from build123d import *

# Parameters (mm, degrees)
SKETCH1_W           = 111.5
SKETCH1_H           = 75
BOSS_EXTRUDE1_DEPTH = 63
CUT_EXTRUDE1_REACH  = 114.703
SKETCH3_W           = 22
SKETCH3_H           = 7
CUT_EXTRUDE2_DEPTH  = 15
CUT_EXTRUDE3_DEPTH  = 15
FILLET1_R           = 10
FILLET2_R           = 2


with BuildPart() as part:
    # Sketch1 → Boss-Extrude1 (new body)
    with BuildSketch(Plane(origin=(0, 0, 0), x_dir=(1, 0, 0), z_dir=(0, 1, 0))):
        Rectangle(SKETCH1_W, SKETCH1_H)
    extrude(amount=BOSS_EXTRUDE1_DEPTH)

    # Sketch2 → Cut-Extrude1 (cut, up to next)
    with BuildSketch(Plane.XY.offset(37.5), mode=Mode.PRIVATE) as cut_extrude1_sk1:
        Polygon((-55.75, 41), (-33.75, 63), (-55.75, 63), align=None)
    cut_extrude1_tool1 = extrude(cut_extrude1_sk1.sketch, amount=-CUT_EXTRUDE1_REACH, mode=Mode.PRIVATE) & part.part
    # Sketch2 → Cut-Extrude1 (cut, up to next)
    with BuildSketch(Plane.XY.offset(37.5), mode=Mode.PRIVATE) as cut_extrude1_sk2:
        Polygon((-55.75, 15), (-40.75, 0), (-55.75, 0), align=None)
    cut_extrude1_tool2 = extrude(cut_extrude1_sk2.sketch, amount=-CUT_EXTRUDE1_REACH, mode=Mode.PRIVATE) & part.part
    add(cut_extrude1_tool1.solids().sort_by_distance((-48.416667, 55.666667, 37.5))[0], mode=Mode.SUBTRACT)
    add(cut_extrude1_tool2.solids().sort_by_distance((-50.75, 5, 37.5))[0], mode=Mode.SUBTRACT)

    # Sketch3 → Cut-Extrude2 (cut)
    with BuildSketch(Plane(origin=(0, 63, 0), x_dir=(1, 0, 0), z_dir=(0, 1, 0))):
        Polygon((31.25, -30.5), (-33.75, -30.5), (-33.75, -37.5), (55.75, -37.5), (55.75, 37.5), (-33.75, 37.5), (-33.75, 30.5), (31.25, 30.5), align=None)
        with Locations((-44.75, -34)):
            Rectangle(SKETCH3_W, SKETCH3_H)
        with Locations((-44.75, 34)):
            Rectangle(SKETCH3_W, SKETCH3_H)
    extrude(amount=-CUT_EXTRUDE2_DEPTH, mode=Mode.SUBTRACT)

    # Sketch4 → Cut-Extrude3 (cut, symmetric)
    with BuildSketch(Plane.XY):
        Polygon((-53.628679656, 43.121320344), (-38.699747468, 58.050252532), (-38.699747468, 55.221825407), (-50.800252532, 43.121320344), align=None)
    extrude(amount=CUT_EXTRUDE3_DEPTH, both=True, mode=Mode.SUBTRACT)

    # Fillet1
    # the kernel refuses this fillet: 10 mm, written as the material it takes off along each edge
    with BuildSketch(Plane(origin=(-55.75, 41, 47.855339059), x_dir=(0.7071067811865432, 0.7071067811865519, 0), z_dir=(0, 0, -1)), Plane(origin=(-40.75, 0, 47.855339059), x_dir=(-0.707106781186546, 0.707106781186549, 0), z_dir=(0, 0, -1))) as fillet1_piece_1:
        with BuildLine():
            CenterArc((FILLET1_R * 0.414213562373, FILLET1_R), FILLET1_R, 225, 45)
            Line((-FILLET1_R * 0.292893218813, FILLET1_R * 0.292893218813), (0, 0))
            Line((0, 0), (FILLET1_R * 0.414213562373, 0))
        make_face()
    extrude(amount=95.710678119, mode=Mode.SUBTRACT)
    with BuildSketch(Plane(origin=(-55.75, 15, 47.855339059), x_dir=(0.7071067811865466, -0.7071067811865482, 0), z_dir=(0, 0, -1))) as fillet1_piece_2:
        with BuildLine():
            CenterArc((FILLET1_R * 0.414213562373, -FILLET1_R), FILLET1_R, 90, 45)
            Line((-FILLET1_R * 0.292893218813, -FILLET1_R * 0.292893218813), (0, 0))
            Line((0, 0), (FILLET1_R * 0.414213562373, 0))
        make_face()
    extrude(amount=95.710678119, mode=Mode.SUBTRACT)
    with BuildSketch(Plane(origin=(55.75, 0, -62.5), x_dir=(-1, 0, 0), z_dir=(0, 0, 1))) as fillet1_piece_3:
        with BuildLine():
            CenterArc((FILLET1_R, -FILLET1_R), FILLET1_R, 90, 90)
            Line((0, -FILLET1_R), (0, 0))
            Line((0, 0), (FILLET1_R, 0))
        make_face()
    extrude(amount=125, mode=Mode.SUBTRACT)

    # Fillet2
    fillet2_edges = [part.edges().sort_by_distance(p)[0] for p in [
        (4.571067812, 0, -37.5),
        (-48.25, 7.5, -37.5),
        (52.821067812, 2.928932188, -37.5),
        (-40.4346987, 0.761204675, -37.5),
        (-54.988795325, 15.3153013, -37.5),
        (-54.988795325, 40.6846987, -37.5),
        (-50.785533906, 45.964466094, -37.5),
        (55.75, 29, 37.5),
        (55.75, 29, -37.5),
        (3.5, 48, -37.5),
        (3.5, 48, 37.5),
        (55.75, 48, 0),
        (-50.785533906, 45.964466094, 37.5),
        (-55.75, 28, 37.5),
        (-48.25, 7.5, 37.5),
        (4.571067812, 0, 37.5),
        (52.821067812, 2.928932188, 37.5),
        (-40.4346987, 0.761204675, 37.5),
        (-54.988795325, 15.3153013, 37.5),
        (-54.988795325, 40.6846987, 37.5),
        (-55.75, 28, -37.5),
    ]]
    fillet(fillet2_edges, radius=FILLET2_R)


solid = part.part
Model file for the job. Use its own axes, mm. A direction names the side the tool comes from. Coordinates: 2 decimals unless noted, no trailing zeros. Write each loop counter-clockwise with the first axis right and the second up, starting at its lowest first coordinate (ties: lowest second). Pieces come first, ordered by that corner, then holes. Notation, with made-up numbers: (39.25, 65) -> (43.25, 65) arc R22 ccw to (43.25, 100) -> close; hole circle Ø11 at (42.25, 4.25). An arc over 180 degrees is marked (long way). One line per item, written item: value. Start each with the question number.
1) Slice it at C-C on z = 4. Write the cut outline in (x, y).
2) Pull direction Z, two halves, no side cores. Call faces 1 (the face through (-44.665, 49.256, 0.21)), 2 (the face through (-37.06, 59.69, 0.5)), 3 (the face through (-47.76, 7.86, 36.93)): +Z half, -Z half, draft (parallel to the pull), parting line (faces both ways), or undercut.
3) Probe probe 1 along Y at (x, z) = (28, 31.5); probe 2 along X at (y, z) = (37.5, 20); probe 3 along X at (y, z) = (50, -1.5). List the from-to ranges inside material, lowest first.
4) Which spindle directions (+Z, -Z, +X, -X, +Y, -Y) get a long thin tool onto all of the face, cutting with end or side? Do faces 4 (the face through (-48.31, 7.56, 0.5)), 5 (the face through (-9, 56, -30.5)), 6 (the face through (-55.01, 40.63, 0.5)), 7 (the face through (-52, 43.121, 0)), 8 (the face through (31.25, 56, 0)). Say none if no direction does.
5) Slice it at A-A on z = -23. Write the cut outline in (x, y).
6) Slice it at B-B on x = 12. Write the cut outline in (y, z).
7) Flat gauge pins, fed straight in: pin 1 Ø12 at (x, y) = (-22, 55) entering from +Z; pin 2 Ø1.5 at (y, z) = (47, -19) entering from -X; pin 3 Ø1.4 at (y, z) = (57.5, -2) entering from -X; pin 4 Ø12 at (x, y) = (-47.5, 47.5) entering from -Z. Where does each tip first touch, or does it go through?
Answers follow:
1. outline: (-55.75, 19.14) arc R10 ccw to (-52.82, 12.07) -> (-43.68, 2.93) arc R10 ccw to (-36.61, 0) -> (45.75, 0) arc R10 ccw to (55.75, 10) -> (55.75, 46) arc R2 ccw to (53.75, 48) -> (31.25, 48) -> (31.25, 63) -> (-33.75, 63) -> (-38.7, 58.05) -> (-38.7, 55.22) -> (-50.8, 43.12) -> (-53.55, 43.12) arc R10 ccw to (-55.75, 36.86) -> close
2. face 1: undercut
2. face 2: draft
2. face 3: +Z half
3. probe 1: 0 to 48
3. probe 2: -55.73 to 55.75
3. probe 3: -43.92 to 31.25
4. face 4: +Z, -Z, -X, -Y
4. face 5: -Z, +X, -X, +Y
4. face 6: +Z, -Z, -X, +Y
4. face 7: -X, +Y
4. face 8: +Z, -Z, +X, +Y
5. outline: (-55.75, 19.14) arc R10 ccw to (-52.82, 12.07) -> (-43.68, 2.93) arc R10 ccw to (-36.61, 0) -> (45.75, 0) arc R10 ccw to (55.75, 10) -> (55.75, 46) arc R2 ccw to (53.75, 48) -> (31.25, 48) -> (31.25, 63) -> (-33.75, 63) -> (-52.82, 43.93) arc R10 ccw to (-55.75, 36.86) -> close
6. outline: (0, -35.5) arc R2 ccw to (2, -37.5) -> (46, -37.5) arc R2 ccw to (48, -35.5) -> (48, -30.5) -> (63, -30.5) -> (63, 30.5) -> (48, 30.5) -> (48, 35.5) arc R2 ccw to (46, 37.5) -> (2, 37.5) arc R2 ccw to (0, 35.5) -> close
7. pin 1: z = 30.5
7. pin 2: x = -50.5
7. pin 3: x = -38.7
7. pin 4: z = -37.5
